Here's how the part is built. I have some questions about the finished solid (model axes, mm). Round coordinates to 2 decimals unless told otherwise and drop trailing zeros. Loops run counter-clockwise (first coordinate to the right, second up) from the corner with the lowest first, then second, coordinate; pieces in that order, holes last. Notation, with made-up numbers: M -40,80 L 18,80 A22 ccw 18,114 Z; hole C 22,25.25 d8. An arc over 180 degrees is marked long. Answer as CSV lines item,"result".
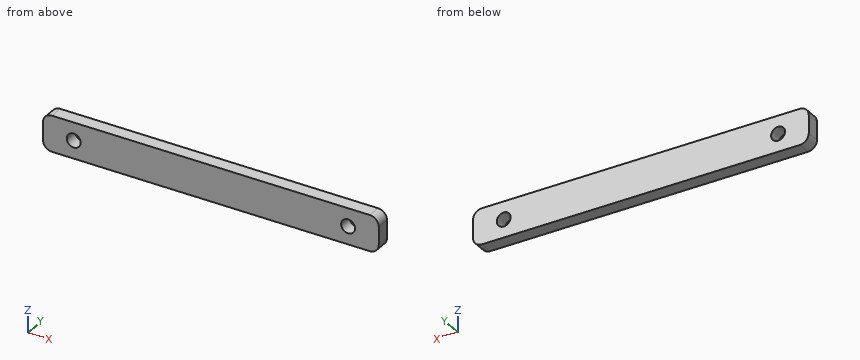
```python
from build123d import *

# Parameters (mm, degrees)
SKETCH_1_W      = 75
SKETCH_1_H      = 8
SKETCH_1_R      = 1.55
EXTRUDE_1_DEPTH = 3
FILLET_1_R      = 2


with BuildPart() as part:
    # 草图1 → 凸台-拉伸1 (new body)
    with BuildSketch(Plane(origin=(0, 0, 0), x_dir=(1, 0, 0), z_dir=(0, 1, 0))):
        Rectangle(SKETCH_1_W, SKETCH_1_H)
        with Locations((-30.645, 0)):
            Circle(SKETCH_1_R, mode=Mode.SUBTRACT)
        with Locations((30.645, 0)):
            Circle(SKETCH_1_R, mode=Mode.SUBTRACT)
    extrude(amount=EXTRUDE_1_DEPTH)

    # 圆角1
    fillet_1_edges = [part.edges().sort_by_distance(p)[0] for p in [
        (-37.5, 1.5, -4),
        (37.5, 1.5, -4),
        (37.5, 1.5, 4),
        (-37.5, 1.5, 4),
    ]]
    fillet(fillet_1_edges, radius=FILLET_1_R)


solid = part.part
```
1. If I drill on line 1 (X direction, y = 0.6, z = 0) (3 decimals); line 2 (X direction, y = 0.35, z = 1); line 3 (X direction, y = 0.9, z = 3), over which ranges is the centre line in solid material (lowest first)? Write a range as [from, to].
Evaluation:
line 1,"x = [-37.5, -32.195], [-29.095, 29.095], [32.195, 37.5]"
line 2,"x = [-37.5, -31.83], [-29.46, 29.46], [31.83, 37.5]"
line 3,"x = [-37.23, 37.23]"
2. I want a section at A-A, the plane z = 0. Please give me the cut outline in (x, y) (3 decimals).
Evaluation:
outline,"M -37.5,0 L -32.195,0 L -32.195,3 L -37.5,3 Z; M -29.095,0 L 29.095,0 L 29.095,3 L -29.095,3 Z; M 32.195,0 L 37.5,0 L 37.5,3 L 32.195,3 Z"
3. I want a section at B-B, the plane y = 1.7. Please give me the cut outline in (x, z) (3 decimals).
Evaluation:
outline,"M -37.5,-2 A2 ccw -35.5,-4 L 35.5,-4 A2 ccw 37.5,-2 L 37.5,2 A2 ccw 35.5,4 L -35.5,4 A2 ccw -37.5,2 Z; hole C -30.645,0 d3.1; hole C 30.645,0 d3.1"
